The listing builds one solid part. Answer for the finished solid, in the listing's coordinates (mm). A direction names the side the tool comes from. Round coordinates to 2 decimals unless told otherwise and drop trailing zeros. Order: outer loops, then holes, each group sorted by start corner. A loop starts at its lowest first (then second) coordinate and runs counter-clockwise, first axis right, second up. Notation, with made-up numbers: (32, 52.25) -> (82, 52.25) arc R18 cw to (82, 80.25) -> close; hole circle Ø6 at (50.5, 43.5). An arc over 180 degrees is marked (long way). Answer in a Markdown table with one row per item. Add a question column.
```python
from build123d import *

# Parameters (mm, degrees)
SKETCH1_R           = 2.6
SKETCH1_R_2         = 9.5
BOSS_EXTRUDE1_DEPTH = 3
SKETCH2_W           = 10
SKETCH2_H           = 3
SKETCH2_W_2         = 3
SKETCH2_H_2         = 10
CUT_EXTRUDE1_DEPTH  = 3


with BuildPart() as part:
    # Sketch1 → Boss-Extrude1 (new body)
    with BuildSketch(Plane(origin=(0, 0, 0), x_dir=(1, 0, 0), z_dir=(0, 1, 0))):
        with BuildLine():
            Line((-32.5, -1.331915835), (-32.5, -34.437048929))
            ThreePointArc((-32.5, -34.437048929), (-24.085532921, -39.90046288), (-17.5, -32.331915835))
            Line((-17.5, -32.331915835), (-17.5, -24.442231617))
            ThreePointArc((-17.5, -24.442231617), (-14.571067812, -17.371163805), (-7.5, -14.442231617))
            Line((-7.5, -14.442231617), (7.5, -14.442231617))
            ThreePointArc((7.5, -14.442231617), (14.571067812, -17.371163805), (17.5, -24.442231617))
            Line((17.5, -24.442231617), (17.5, -32.331915835))
            Line((17.5, -32.331915835), (17.5, -36.417098288))
            ThreePointArc((17.5, -36.417098288), (25.631797985, -41.985078136), (32.5, -34.917098288))
            Line((32.5, -34.917098288), (32.5, -33.831915835))
            Line((32.5, -33.831915835), (32.5, -1.331915835))
            Line((32.5, -1.331915835), (32.5, 3.668084165))
            Line((32.5, 3.668084165), (32.5, 38.668084165))
            Line((32.5, 38.668084165), (32.441371292, 38.668084165))
            Line((32.441371292, 38.668084165), (-6.058628708, 38.668084165))
            Line((-6.058628708, 38.668084165), (-6.058628708, 14.168084165))
            Line((-6.058628708, 14.168084165), (-6.058628708, 11.668084165))
            ThreePointArc((-6.058628708, 11.668084165), (-7.230201584, 8.83965704), (-10.058628708, 7.668084165))
            Line((-10.058628708, 7.668084165), (-28.5, 7.668084165))
            ThreePointArc((-28.5, 7.668084165), (-31.328427125, 6.49651129), (-32.5, 3.668084165))
            Line((-32.5, 3.668084165), (-32.5, 3.101498414))
            Line((-32.5, 3.101498414), (-32.5, -1.331915835))
        make_face()
        with Locations(Location((-25, -32.331915835, 0), (0, 0, 270))):
            Circle(SKETCH1_R, mode=Mode.SUBTRACT)
        with Locations(Location((25, -32.331915835, 0), (0, 0, 270))):
            Circle(SKETCH1_R, mode=Mode.SUBTRACT)
        with Locations(Location((13.245823136, 23.897996209, 0), (0, 0, 270))):
            Circle(SKETCH1_R_2, mode=Mode.SUBTRACT)
    extrude(amount=BOSS_EXTRUDE1_DEPTH)

    # Sketch2 → Cut-Extrude1 (cut)
    with BuildSketch(Plane(origin=(0, 3, 0), x_dir=(1, 0, 0), z_dir=(0, 1, 0))):
        with Locations((4.470685646, 37.168084165)):
            Rectangle(SKETCH2_W, SKETCH2_H)
        with Locations((-4.558628708, 23.22062572)):
            Rectangle(SKETCH2_W_2, SKETCH2_H_2)
        with Locations((21.970685646, 37.168084165)):
            Rectangle(SKETCH2_W, SKETCH2_H)
        with Locations((31, 23.22062572)):
            Rectangle(SKETCH2_W_2, SKETCH2_H_2)
    extrude(amount=-CUT_EXTRUDE1_DEPTH, mode=Mode.SUBTRACT)


solid = part.part
```
Item 1: For a pull along X with two mould halves and no side action, classify faces 4 (the face through (-6.059, 1, -15)), 5 (the face through (7, 0, 1)), 6 (the face through (17.5, 1, 30)) as released by +X, released by -X, zero draft, split by the parting line, or undercut.
Item 2: The part is cut by section D-D, the plane z = -10. Give the vertices of the cut face in (x, y), and give its area (3 significant figures).
Item 3: A tool of negligible diameter and unlimited length cuts with its end or side. For faces 1 (the face through (29.5, 2, -23)), 2 (the face through (-17.5, 1, 28)), 3 (the face through (-0.529, 2, -37)), from which of +Z, -Z, +X, -X, +Y, -Y can it reach the whole face along a straight path? Write none if from no direction.
Item 4: The part is cut by section A-A, the plane z = 26. Give the vertices of the cut face in (x, y).
Item 5: The part is cut by section C-C, the plane y = 1.4. State how many separate pieces and enclosed holes the cut face has, and give its area (3 significant figures).
Item 6: Find the intervals of material crossed by probe 1 along Z at (x, y) = (7, 0.7); probe 2 along X at (y, z) = (2.25, -13.5); probe 3 along X at (y, z) = (2.25, 33), in increasing order. Write a range as [from, to].
Item 7: The part is cut by section B-B, the plane x = 25. Give the vertices of the cut face in (y, z), and give its area (3 significant figures).
Item 8: Flat-ended cylindrical pins translate along their axes: P1, Ø1.5, axis at x = -4.5, y = 2, coming from the +Z side; P2, Ø4, axis at x = -25, z = 32.33, coming from the -Y side; P3, Ø0.9, axis at x = 4, y = 1.5, coming from the -Z side; P4, Ø1.5, axis at x = 31.5, y = 1.5, coming from the +Z side. Find the tip coordinate at first contact, or state that the pin passes through.
Resolved:
| question | item | result |
|---|---|---|
| 1 | face 4 | released by -X |
| 1 | face 5 | zero draft |
| 1 | face 6 | undercut |
| 2 | outline | (-6.42, 0) -> (32.5, 0) -> (32.5, 3) -> (-6.42, 3) -> close |
| 2 | area | 117 mm2 |
| 3 | face 1 | +X, +Y, -Y |
| 3 | face 2 | +Z, +Y, -Y |
| 3 | face 3 | -Z, +Y, -Y |
| 4 | outline | (-32.5, 0) -> (-17.5, 0) -> (-17.5, 3) -> (-32.5, 3) -> close; (17.5, 0) -> (32.5, 0) -> (32.5, 3) -> (17.5, 3) -> close |
| 5 | separate pieces | 1 |
| 5 | enclosed holes | 3 |
| 5 | area | 2,980 mm2 |
| 6 | probe 1 | [-35.67, -31.06], [-16.74, 14.44] |
| 6 | probe 2 | [-6.06, 32.5] |
| 6 | probe 3 | [-32.5, -27.51], [-22.49, -17.53], [17.5, 22.49], [27.51, 32.5] |
| 7 | outline | (0, -35.67) -> (3, -35.67) -> (3, 29.73) -> (0, 29.73) -> close; (0, 34.93) -> (3, 34.93) -> (3, 42.02) -> (0, 42.02) -> close |
| 7 | area | 217 mm2 |
| 8 | P1 | z = 14.44 |
| 8 | P2 | through |
| 8 | P3 | z = -35.67 |
| 8 | P4 | z = 39.27 |
